CAD build for the part. Positions are in the model's coordinates, mm. Give positions to 0.01 mm unless a question says otherwise; leave off trailing zeros. Loops run counter-clockwise (first coordinate to the right, second up) from the corner with the lowest first, then second, coordinate; pieces in that order, holes last. Notation, with made-up numbers: (14, 67) -> (25, 67) arc R27 cw to (25, 85) -> close; hole circle Ø11 at (48.25, -18). An arc over 180 degrees is marked (long way). Write each question's results on one line, items separated by ' | '. Start each with the question number.
```python
from build123d import *

# Parameters (mm, degrees)
F0_W     = 500
F0_H     = 320
F1_DEPTH = 15.88
F2_W     = 15.88
F2_H     = 7.94
F3_DEPTH = 320.001
F4_W     = 7.94
F4_H     = 15.88
F5_DEPTH = 484.121
F6_R     = 7.5


with BuildPart() as f1:
    # F0 (on Front) → F1 (new body)
    with BuildSketch(Plane.XZ):
        with Locations((276.000002, -4e-06)):
            Rectangle(F0_W, F0_H)
        with BuildLine():
            ThreePointArc((376.000002, -85.000004), (368.677672, -102.677673), (351.000002, -110.000004))
            Line((351.000002, -110.000004), (201.000002, -110.000004))
            ThreePointArc((201.000002, -110.000004), (176.000002, -85.000004), (201.000002, -60.000004))
            Line((201.000002, -60.000004), (351.000002, -60.000004))
            ThreePointArc((351.000002, -60.000004), (368.677672, -67.322334), (376.000002, -85.000004))
        make_face(mode=Mode.SUBTRACT)
    extrude(amount=F1_DEPTH)

    # F2 (on face) → F3 (cut, through all)
    with BuildSketch(Plane(origin=(0, 0, -160.000004), x_dir=(1, 0, 0), z_dir=(0, 0, -1))):
        with Locations((33.940002, 11.91)):
            Rectangle(F2_W, F2_H)
        with Locations((518.060002, 11.91)):
            Rectangle(F2_W, F2_H)
    extrude(amount=-F3_DEPTH, mode=Mode.SUBTRACT)

    # F4 (on face) → F5 (cut, through all)
    with BuildSketch(Plane(origin=(41.880002, 0, 0), x_dir=(0, -1, 0), z_dir=(-1, 0, 0))):
        with Locations((11.91, 152.059996)):
            Rectangle(F4_W, F4_H)
    extrude(amount=-F5_DEPTH, mode=Mode.SUBTRACT)

    # F6
    f6_edges = [f1.edges().sort_by_distance(p)[0] for p in [
        (276.000002, 0, -60.000004),
        (276.000002, -15.88, -60.000004),
    ]]
    fillet(f6_edges, radius=F6_R)


solid = f1.part
```
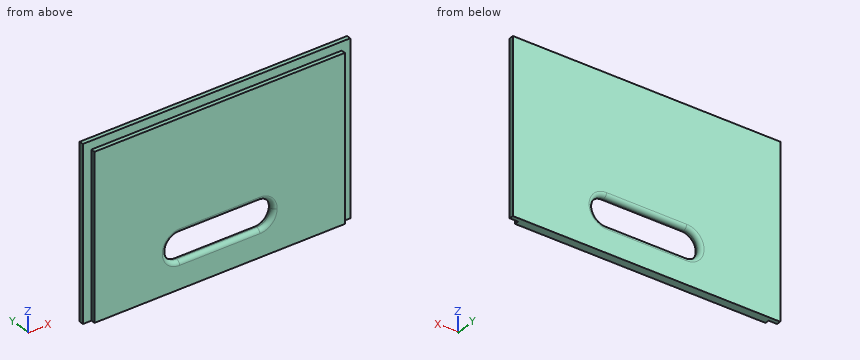
Q1. Saw through at C-C, the plane z = 33. List the corners of the cut face in (x, y).
Q2. Saw through at A-A, the plane x = 257. List the corners of the cut face in (y, z).
Q3. Wall check: L1, parallel to Z at x = 460.5, y = -13.5; L2, parallel to X at y = -14, z = -139; L3, parallel to Z at x = 182.5, y = -4. Give the ranges that are in metal, low to high.
Q4. Drop flat-ended pins along their axis: pin 1 (1.5 mm diameter, centred on x = 126, y = -8.5, fed in from +Z); pin 2 (6.5 mm diameter, centred on y = -12.5, z = 43, fed in from -X); pin 3 (4 mm diameter, centred on x = 163.5, y = -13.5, fed in from +Z); pin 4 (1.5 mm diameter, centred on y = -12.5, z = -12.5, fed in from +X). Give the stop position or say it passes through.
Q5. Saw through at B-B, the plane y = -11. List the corners of the cut face in (x, z), then the cut area to 3 significant figures.
Q6. Saw through at D-D, the plane x = 417. List the corners of the cut face in (y, z), then the cut area to 3 significant figures.
Answer block:
1) outline: (26, -7.94) -> (41.88, -7.94) -> (41.88, -15.88) -> (510.12, -15.88) -> (510.12, -7.94) -> (526, -7.94) -> (526, 0) -> (26, 0) -> close
2) outline: (-15.88, -160) -> (0, -160) -> (0, -117.5) arc R7.5 ccw to (-7.5, -110) -> (-8.38, -110) arc R7.5 ccw to (-15.88, -117.5) -> close; (-15.88, -52.5) arc R7.5 ccw to (-8.38, -60) -> (-7.5, -60) arc R7.5 ccw to (0, -52.5) -> (0, 160) -> (-7.94, 160) -> (-7.94, 144.12) -> (-15.88, 144.12) -> close
3) L1: z = -160 to 144.12 | L2: x = 41.88 to 510.12 | L3: z = -160 to -103.08, -66.92 to 160
4) pin 1: stops at z = 160 | pin 2: stops at x = 41.88 | pin 3: stops at z = 144.12 | pin 4: stops at x = 510.12
5) outline: (41.88, -160) -> (510.12, -160) -> (510.12, 144.12) -> (41.88, 144.12) -> close; hole (201, -110.47) -> (351, -110.47) arc R25.47 ccw to (376.47, -85) arc R25.47 ccw to (351, -59.53) -> (201, -59.53) arc R25.47 ccw to start | area: 133,000 mm2
6) outline: (-15.88, -160) -> (0, -160) -> (0, 160) -> (-7.94, 160) -> (-7.94, 144.12) -> (-15.88, 144.12) -> close | area: 4,960 mm2
